Work out the finished part from the listing and answer in its coordinate system (mm). Face numbers are marked on the shaded views. A direction names the side the tool comes from. Coordinates: 2 decimals unless noted, no trailing zeros. Order: outer loops, then holes, each group sorted by start corner. A loop starts at its lowest first (then second) coordinate and runs counter-clockwise, first axis right, second up. Notation, with made-up numbers: M 42,0 L 93,0 A18 cw 93,7 Z; hole C 75.5,-27.5 d1. An arc over 180 degrees is marked long. Use a Markdown table: item, result.
from build123d import *

# Parameters (mm, degrees)
EXTRUSION4_DEPTH = 25.4


with BuildPart() as part:
    # Sketch1 → Extrusion4 (new body)
    with BuildSketch(Plane.XY):
        with BuildLine():
            Line((-14.999999918, 14.999999985), (-4.099998388, 14.999999985))
            Line((-4.099998388, 14.999999985), (-4.099998388, 12.499999985))
            Line((-4.099998388, 12.499999985), (-6.799995338, 12.499999985))
            Line((-6.799995338, 12.499999985), (-6.799995338, 7.860655585))
            Line((-6.799995338, 7.860655585), (-3.941497908, 5.002158155))
            Line((-3.941497908, 5.002158155), (3.941498082, 5.002158155))
            Line((3.941498082, 5.002158155), (6.799995512, 7.860655585))
            Line((6.799995512, 7.860655585), (6.799995512, 12.499999985))
            Line((6.799995512, 12.499999985), (4.099998562, 12.499999985))
            Line((4.099998562, 12.499999985), (4.099998562, 14.999999985))
            Line((4.099998562, 14.999999985), (14.810114901, 14.999999985))
            Line((14.810114901, 14.999999985), (14.858211116, 11.334807121))
            ThreePointArc((14.858211116, 11.334807121), (10.399126577, -6.225213544), (-2.242564242, -19.203095263))
            Line((-2.242564242, -19.203095263), (-5.213160142, -20.9705416))
            Line((-5.213160142, -20.9705416), (-10.940381729, -11.050702829))
            Line((-10.940381729, -11.050702829), (-8.775318226, -9.800702836))
            Line((-8.775318226, -9.800702836), (-7.425319757, -12.138968783))
            Line((-7.425319757, -12.138968783), (-3.407529648, -9.819296585))
            Line((-3.407529648, -9.819296585), (-2.361246978, -5.914516485))
            Line((-2.361246978, -5.914516485), (-6.302744968, 0.912358295))
            Line((-6.302744968, 0.912358295), (-10.207525068, 1.958640965))
            Line((-10.207525068, 1.958640965), (-14.225315169, -0.361031229))
            Line((-14.225315169, -0.361031229), (-12.875316699, -2.699297177))
            Line((-12.875316699, -2.699297177), (-15.040380206, -3.949297173))
            Line((-15.040380206, -3.949297173), (-20.490380962, 5.490381032))
            Line((-20.490380962, 5.490381032), (-17.499999918, 7.216878355))
            ThreePointArc((-17.499999918, 7.216878355), (-15.669872899, 9.047005374), (-14.999999918, 11.547005375))
            Line((-14.999999918, 11.547005375), (-14.999999918, 14.999999985))
        make_face()
        with BuildLine():
            Line((-3.803644053, 2.604283261), (-2.920581563, 2.840899141))
            Line((-2.920581563, 2.840899141), (-2.821802903, 2.783869251))
            ThreePointArc((-2.821802903, 2.783869251), (-2.642326542, 2.745128481), (-2.473891573, 2.818219331))
            ThreePointArc((-2.473891573, 2.818219331), (-0.48947315, 3.717918241), (1.660187067, 3.362481111))
            ThreePointArc((1.660187067, 3.362481111), (1.841800057, 3.335474951), (2.005134057, 3.419347561))
            Line((2.005134057, 3.419347561), (2.085786497, 3.500000001))
            Line((2.085786497, 3.500000001), (3.000000057, 3.500000001))
            ThreePointArc((3.000000057, 3.500000001), (3.353553447, 3.353553391), (3.500000057, 3.000000001))
            Line((3.500000057, 3.000000001), (3.500000057, 2.085786441))
            Line((3.500000057, 2.085786441), (3.419347617, 2.005134001))
            ThreePointArc((3.419347617, 2.005134001), (3.335475004, 1.841799992), (3.362481172, 1.660186995))
            ThreePointArc((3.362481172, 1.660186995), (3.247595339, -1.874999996), (0.243476512, -3.742087545))
            ThreePointArc((0.243476512, -3.742087545), (0.072691963, -3.809506014), (-0.026823118, -3.963808835))
            Line((-0.026823118, -3.963808835), (-0.056343958, -4.073982115))
            Line((-0.056343958, -4.073982115), (-0.848076128, -4.531088895))
            ThreePointArc((-0.848076128, -4.531088895), (-1.227485649, -4.581039105), (-1.531088828, -4.348076195))
            Line((-1.531088828, -4.348076195), (-1.988195608, -3.556344025))
            Line((-1.988195608, -3.556344025), (-1.958674768, -3.446170745))
            ThreePointArc((-1.958674768, -3.446170745), (-1.967705959, -3.262783044), (-2.081900468, -3.119004655))
            ThreePointArc((-2.081900468, -3.119004655), (-3.464548158, -1.435062862), (-3.677595258, 0.733343355))
            ThreePointArc((-3.677595258, 0.733343355), (-3.698514209, 0.915757746), (-3.821802888, 1.051818445))
            Line((-3.821802888, 1.051818445), (-3.920581548, 1.108848335))
            Line((-3.920581548, 1.108848335), (-4.157197428, 1.991910825))
            ThreePointArc((-4.157197428, 1.991910825), (-4.10724722, 2.371320342), (-3.803644053, 2.604283261))
        make_face(mode=Mode.SUBTRACT)
        with BuildLine():
            Line((-13.999999918, 11.547005365), (-13.999999918, 13.999999985))
            Line((-13.999999918, 13.999999985), (-7.799995348, 13.999999985))
            Line((-7.799995348, 13.999999985), (-7.799995348, 7.567762365))
            ThreePointArc((-7.799995348, 7.567762365), (-7.647754416, 6.802395499), (-7.214208908, 6.153548805))
            Line((-7.214208908, 6.153548805), (-5.676298958, 4.615638855))
            ThreePointArc((-5.676298958, 4.615638855), (-5.485596608, 3.167110716), (-6.835409948, 2.607999725))
            Line((-6.835409948, 2.607999725), (-8.936234008, 3.170913835))
            ThreePointArc((-8.936234008, 3.170913835), (-9.714924484, 3.221951904), (-10.453872098, 2.971112985))
            Line((-10.453872098, 2.971112985), (-16.024353279, -0.245005824))
            Line((-16.024353279, -0.245005824), (-19.124355567, 5.124355624))
            Line((-19.124355567, 5.124355624), (-16.999999918, 6.350852945))
            ThreePointArc((-16.999999918, 6.350852945), (-14.803847494, 8.547005366), (-13.999999918, 11.547005365))
        make_face(mode=Mode.SUBTRACT)
        with BuildLine():
            Line((7.799995502, 7.567762365), (7.799995491, 13.999999985))
            Line((7.799995491, 13.999999985), (14.000000062, 13.999999985))
            Line((14.000000062, 13.999999985), (14.000000062, 11.547005385))
            ThreePointArc((14.000000062, 11.547005385), (12.9999649, 3.361510856), (10.058687082, -4.342467065))
            ThreePointArc((10.058687082, -4.342467065), (9.755046631, -4.589262395), (9.366647572, -4.541811055))
            Line((9.366647572, -4.541811055), (5.235555602, -2.156723995))
            ThreePointArc((5.235555602, -2.156723995), (5.019640061, -1.905157444), (5.008550772, -1.573823355))
            ThreePointArc((5.008550772, -1.573823355), (5.247767117, -0.153104957), (5.091786812, 1.279143405))
            ThreePointArc((5.091786812, 1.279143405), (5.115772962, 3.319255937), (6.142816242, 5.082155985))
            Line((6.142816242, 5.082155985), (7.214209062, 6.153548805))
            ThreePointArc((7.214209062, 6.153548805), (7.647754561, 6.802395503), (7.799995502, 7.567762365))
        make_face(mode=Mode.SUBTRACT)
        with BuildLine():
            Line((-1.722025028, -9.324462665), (-1.329868038, -7.860912855))
            ThreePointArc((-1.329868038, -7.860912855), (-0.316673452, -6.090017259), (1.438122752, -5.049188375))
            ThreePointArc((1.438122752, -5.049188375), (2.756476373, -4.4681471), (3.867246431, -3.550620473))
            ThreePointArc((3.867246431, -3.550620473), (4.159734815, -3.394557032), (4.485555611, -3.455762103))
            Line((4.485555611, -3.455762103), (8.616647581, -5.840849163))
            ThreePointArc((8.616647581, -5.840849163), (8.851941182, -6.153486949), (8.790030382, -6.539844965))
            ThreePointArc((8.790030382, -6.539844965), (3.588828705, -12.939055237), (-2.999999918, -17.897858355))
            Line((-2.999999918, -17.897858355), (-5.124355566, -19.12435565))
            Line((-5.124355566, -19.12435565), (-8.224357859, -13.754994194))
            Line((-8.224357859, -13.754994194), (-2.653876678, -10.538875385))
            ThreePointArc((-2.653876678, -10.538875385), (-2.067169998, -10.024347435), (-1.722025028, -9.324462665))
        make_face(mode=Mode.SUBTRACT)
    extrude(amount=EXTRUSION4_DEPTH)


solid = part.part
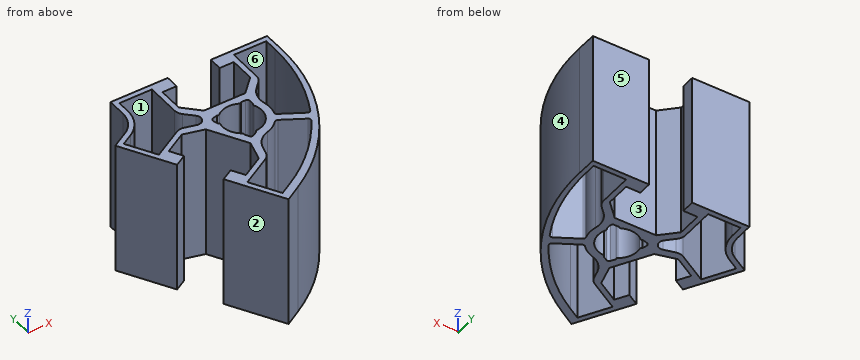
1. Flat-ended cylindrical pins translate along their axes: P1, Ø1.3, axis at x = 5, z = 17, coming from the -Y side; P2, Ø1.7, axis at y = 13, z = 19, coming from the -X side; P3, Ø2, axis at y = 3, z = 12, coming from the +X side. Find the tip coordinate at first contact, or state that the pin passes through.
Answers below:
| item | result |
|---|---|
| P1 | y = -14.13 |
| P2 | x = -15 |
| P3 | x = 14.18 |
2. Find the intervals of material crossed by probe 1 along X at (y, z) = (12, 8.25); probe 2 along Y at (x, z) = (0.5, 8); probe 3 along X at (y, z) = (13, 18), in increasing order.
Answers below:
| item | result |
|---|---|
| probe 1 | -15 to -14, -7.8 to -6.8, 6.8 to 7.8, 14 to 14.85 |
| probe 2 | -17.39 to -15.58, -5.45 to -3.72, 3.72 to 5 |
| probe 3 | -15 to -14, -7.8 to -4.1, 4.1 to 7.8, 14 to 14.84 |
3. For the marked faces 1, 2 and 3, determine the directions among +Z, -Z, +X, -X, +Y, -Y from which every point of the face is accessible in a straight line to the end or side of a thin tool.
Answers below:
| item | result |
|---|---|
| face 1 | +Z, -Z |
| face 2 | +Z, -Z, -X, -Y |
| face 3 | +Z, -Z, +Y |
4. Section D-D on z = 18 is taken. Give the number of separate pieces and of enclosed holes in the cut face, then the cut area to 3 significant figures.
Answers below:
| item | result |
|---|---|
| separate pieces | 1 |
| enclosed holes | 4 |
| area | 231 mm² |
5. Section C-C on y = 10.5 is taken. Determine the outline of the cut face in (x, z).
Answers below:
| item | result |
|---|---|
| outline | M -15.11,0 L -14.09,0 L -14.09,25.4 L -15.11,25.4 Z; M -7.8,0 L -6.8,0 L -6.8,25.4 L -7.8,25.4 Z; M 6.8,0 L 7.8,0 L 7.8,25.4 L 6.8,25.4 Z; M 13.98,0 L 14.86,0 L 14.86,25.4 L 13.98,25.4 Z |
6. Section A-A on y = -7 is taken. Determine the outline of the cut face in (x, z), then the cut area to 3 significant figures.
Answers below:
| item | result |
|---|---|
| outline | M -2.65,0 L -0.99,0 L -0.99,25.4 L -2.65,25.4 Z; M 8.5,0 L 9.95,0 L 9.95,25.4 L 8.5,25.4 Z |
| area | 79.3 mm² |
7. For a pull along X with two mould halves and no side action, classify the marked faces 4, 5 and 6 as +X half, -X half, draft (parallel to the pull), parting line (faces both ways), or undercut.
Answers below:
| item | result |
|---|---|
| face 4 | +X half |
| face 5 | draft |
| face 6 | undercut |
8. Section B-B on x = 12.5 is taken. Determine the outline of the cut face in (y, z), then the cut area to 3 significant figures.
Answers below:
| item | result |
|---|---|
| outline | M -1.76,0 L 1.56,0 L 1.56,25.4 L -1.76,25.4 Z; M 14,0 L 15,0 L 15,25.4 L 14,25.4 Z |
| area | 110 mm² |
